Autodesk Inventor part; units mm, degrees
ref_plane "YZ Plane" through (0, 0, 0) normal (1, 0, 0) x (0, 1, 0)
ref_plane "XZ Plane" through (0, 0, 0) normal (0, 1, 0) x (-1, 0, 0)
ref_plane "XY Plane" through (0, 0, 0) normal (0, 0, 1) x (1, 0, 0)
sketch "Эскиз1" plane through (0, 0, 0) normal (1, 0, 0) x (0, 1, 0)
  circle A0 centre (0, 0) radius 1.5
  dimension "d0" = 3
extrude "Выдавливание1" add sketch "Эскиз1" along normal blind 10
sketch "Эскиз2" plane through (10, 0, 0) normal (1, 0, 0) x (0, 0, -1)
  circle A0 centre (0, 0.9066) radius 0.3125
  circle A1 centre (0, -0.9266) radius 0.357
  point P0 (0, 0)
extrude "Выдавливание2" add sketch "Эскиз2" along normal blind 4
chamfer "Фаска1" distance 0.2 angle 45 2 edges at (10, -1.5, 0) (0, -1.5, 0)
properties part number "термодатчик1"
Input: part model. Units: mm. Frame: model coordinates. A direction names the side the tool comes from. Give positions to 0.01 mm unless a question says otherwise; leave off trailing zeros. Loops run counter-clockwise (first coordinate to the right, second up) from the corner with the lowest first, then second, coordinate; pieces in that order, holes last. Notation, with made-up numbers: M 87.25,67 L 112.25,67 A28 cw 112.25,94 Z; hole C 66,22.25 d9. An arc over 180 degrees is marked long. Answer as CSV lines item,"result". Start each with the question number.
1. Line query: L1, parallel to X at y = -0.05, z = -0.6; L2, parallel to Y at x = 8, z = 0.75; L3, parallel to Z at x = 3.75, y = -1.15. Output: solid intervals per line, ascending.
2. Pin query (flat end, axial travel): P1, Ø0.8, axis at y = 0, z = 0.5, coming from the +X side; P2, Ø1, axis at x = 4, y = 1, coming from the +Z side; P3, Ø1, axis at x = 7, z = 1, coming from the +Y side. Return the tip coordinate at first contact, or that it passes through.
3. Section C-C on x = 9.5. Return loops of the section in (y, z), plus the area to 3 significant figures.
4. Reachability of faces 1 (the face through (0, 0, 0)), 2 (the face through (10, 0, 0)) from +Z, -Z, +X, -X, +Y, -Y: full face, straight path, thin tool, end or side. Return the list, or none.
5. Section B-B on y = 0. Return loops of the section in (x, z).
Computed values:
1,L1,"x = 0 to 10"
1,L2,"y = -1.3 to 1.3"
1,L3,"z = -0.96 to 0.96"
2,P1,"stops at x = 10"
2,P2,"stops at z = 1.41"
2,P3,"stops at y = 1.41"
3,outline,"C 0,0 d3"
3,area,"7.07 mm²"
4,face 1,"+Z, -Z, -X, +Y, -Y"
4,face 2,"+X"
5,outline,"M 0,-1.3 L 0.2,-1.5 L 9.8,-1.5 L 10,-1.3 L 10,1.3 L 9.8,1.5 L 0.2,1.5 L 0,1.3 Z"
